Model file for the job. Use its own axes, mm. Face numbers are marked on the shaded views. A direction names the side the tool comes from. Coordinates: 2 decimals unless noted, no trailing zeros. Write each loop counter-clockwise with the first axis right and the second up, starting at its lowest first coordinate (ties: lowest second). Pieces come first, ordered by that corner, then holes. Notation, with made-up numbers: (87, -22.75) - (108, -22.75) arc R15 ccw to (108, 1.25) - close; hole circle Ø11 at (4, 34.5). An arc over 180 degrees is marked (long way). Put each result on its own line as item: value. Start each with the question number.
1. Drill centre lines: L1, parallel to X at y = 10.5, z = -0.25; L2, parallel to X at y = 24, z = 2.5; L3, parallel to Y at x = 4.5, z = -7. Where is each one in solid material? Low to high. Write a range as from..to.
2. Saw through at B-B, the plane x = 0. Write the cut outline in (y, z), plus the area to 3 significant figures.
3. Which spindle directions (+Z, -Z, +X, -X, +Y, -Y) get a long thin tool onto all of the face, cutting with end or side? Do the marked faces 1 and 2. Say none if no direction does.
4. Saw through at D-D, the plane y = 28. Write the cut outline in (x, z).
5. Saw through at A-A, the plane z = 0. Write the cut outline in (x, y).
6. Drop flat-ended pins along their axis: P1, Ø0.6, axis at x = 4.5, z = 0.5, coming from the +Y side; P2, Ø4, axis at y = 15, z = -9, coming from the +X side; P3, Ø6, axis at y = 25.5, z = -4, coming from the +X side; P4, Ø8, axis at x = -6, y = 11, coming from the -Z side. Give the stop position or say it passes through.
7. Saw through at C-C, the plane y = 18.5. Write the cut outline in (x, z).
```python
from build123d import *

# Parameters (mm, degrees)
CUT_EXTRUDE1_DEPTH      = 36.341194094
CUT_EXTRUDE1_DEPTH_BACK = 36.341194094
SKETCH3_W               = 2
SKETCH3_H               = 2
CHAMFER1_SIZE           = 1


with BuildPart() as part:
    # Sketch2 → Revolve1 (revolve)
    with BuildSketch(Plane.XY):
        Polygon((1, 31), (1, 29), (0, 29), (0, 0), (6, 0), (6, 25), (12, 31), align=None)
    revolve(axis=Axis((0, 0, 0), (0, 1, 0)))

    # Sketch3 → Cut-Extrude1 (cut, two sides: drawn at the far end of the back side and taken through both)
    with BuildSketch(Plane(origin=(0, 0, 0), x_dir=(0, 0, -1), z_dir=(1, 0, 0)).offset(-CUT_EXTRUDE1_DEPTH_BACK)):
        with Locations((0, 30)):
            Rectangle(SKETCH3_W, SKETCH3_H)
    extrude(amount=CUT_EXTRUDE1_DEPTH + CUT_EXTRUDE1_DEPTH_BACK, mode=Mode.SUBTRACT)

    # Chamfer1
    chamfer1_edges = [part.edges().sort_by_distance(p)[0] for p in [
        (-6, 0, 0),
    ]]
    chamfer(chamfer1_edges, length=CHAMFER1_SIZE)


solid = part.part
```
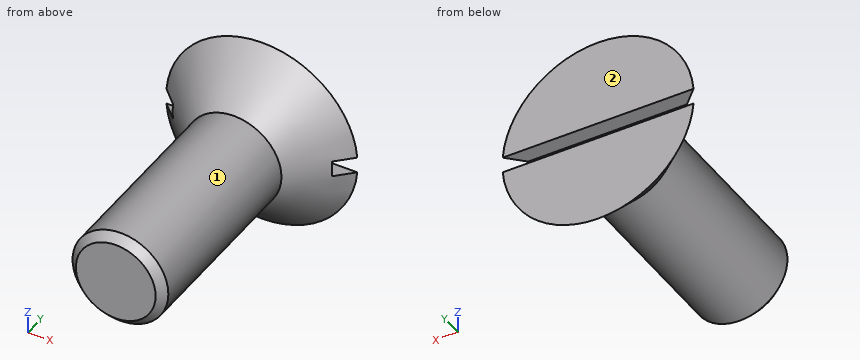
Final values:
1. L1: x = -5.99..5.99
1. L2: x = -5.45..5.45
1. L3: y = 27.32..31
2. outline: (0, -5) - (1, -6) - (25, -6) - (31, -12) - (31, -1) - (29, -1) - (29, 1) - (31, 1) - (31, 12) - (25, 6) - (1, 6) - (0, 5) - close
2. area: 403 mm²
3. face 1: -Y
3. face 2: +Z, -Z, +X, -X, +Y
4. outline: circle Ø18 at (0, 0)
5. outline: (-10, 29) - (-6, 25) - (-6, 1) - (-5, 0) - (5, 0) - (6, 1) - (6, 25) - (10, 29) - close
6. P1: stops at y = 29
6. P2: passes through
6. P3: stops at x = 8.83
6. P4: stops at z = -5.66
7. outline: circle Ø12 at (0, 0)
